Geometry: final body of the model. Coordinates: model frame, mm. Face numbers are marked on the shaded views. A direction names the side the tool comes from. Give positions to 0.01 mm unless a question says otherwise; leave off trailing zeros. Order: outer loops, then holes, each group sorted by start corner. A loop starts at its lowest first (then second) coordinate and runs counter-clockwise, first axis right, second up. Notation, with made-up numbers: (62.25, 49.5) - (112.25, 49.5) arc R12 cw to (112.25, 55.5) - close; hole circle Ø9 at (58.25, -20). An arc over 180 degrees is marked (long way). Use one line per item in the form item = value.
from build123d import *

# Parameters (mm, degrees)
SKETCH1_W           = 30
SKETCH1_H           = 85
BOSS_EXTRUDE1_DEPTH = 10
SKETCH2_W           = 30
SKETCH2_H           = 15
BOSS_EXTRUDE2_DEPTH = 2.5
SKETCH3_W           = 3
SKETCH3_H           = 15
BOSS_EXTRUDE3_DEPTH = 3


with BuildPart() as part:
    # Sketch1 → Boss-Extrude1 (new body)
    with BuildSketch(Plane.XY):
        with Locations((15, 42.5)):
            Rectangle(SKETCH1_W, SKETCH1_H)
    extrude(amount=BOSS_EXTRUDE1_DEPTH)

    # Sketch2 → Boss-Extrude2 (add)
    with BuildSketch(Plane.XY.offset(10)):
        with Locations((15, 62.5)):
            Rectangle(SKETCH2_W, SKETCH2_H)
        with Locations((15, 22.5)):
            Rectangle(SKETCH2_W, SKETCH2_H)
    extrude(amount=BOSS_EXTRUDE2_DEPTH)

    # Sketch3 → Boss-Extrude3 (add)
    with BuildSketch(Plane.XY.offset(12.5)):
        with Locations((28.5, 62.5)):
            Rectangle(SKETCH3_W, SKETCH3_H)
        with Locations((28.5, 22.5)):
            Rectangle(SKETCH3_W, SKETCH3_H)
        with Locations((1.5, 22.5)):
            Rectangle(SKETCH3_W, SKETCH3_H)
        with Locations((1.5, 62.5)):
            Rectangle(SKETCH3_W, SKETCH3_H)
    extrude(amount=BOSS_EXTRUDE3_DEPTH)


solid = part.part
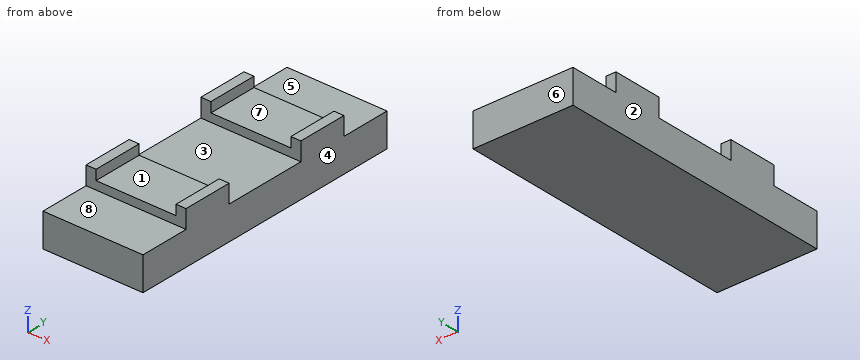
(1) Reachability of the marked faces 4, 5, 6, 7 and 8 from +Z, -Z, +X, -X, +Y, -Y: full face, straight path, thin tool, end or side. Return the list, or none.
Computed values:
face_4 = +Z, -Z, +X, +Y, -Y
face_5 = +Z, +X, -X, +Y
face_6 = +Z, -Z, +X, -X, +Y
face_7 = +Z, +Y, -Y
face_8 = +Z, +X, -X, -Y
(2) Cut plane B-B on y = 56. Output: boundary loops of the cut face in (x, z).
Computed values:
outline = (0, 0) - (30, 0) - (30, 15.5) - (27, 15.5) - (27, 12.5) - (3, 12.5) - (3, 15.5) - (0, 15.5) - close
(3) Pull-direction query (X, two-part tool) for the marked faces 1, 2 and 3; classes: released by +X, released by -X, zero draft, split by the parting line, or undercut.
Computed values:
face_1 = undercut
face_2 = released by -X
face_3 = zero draft
(4) Cut plane D-D on x = 28. Output: boundary loops of the cut face in (y, z), plus the area to 4 significant figures.
Computed values:
outline = (0, 0) - (85, 0) - (85, 10) - (70, 10) - (70, 15.5) - (55, 15.5) - (55, 10) - (30, 10) - (30, 15.5) - (15, 15.5) - (15, 10) - (0, 10) - close
area = 1,015 mm²
(5) Cut plane C-C on x = 6.5. Output: boundary loops of the cut face in (y, z).
Computed values:
outline = (0, 0) - (85, 0) - (85, 10) - (70, 10) - (70, 12.5) - (55, 12.5) - (55, 10) - (30, 10) - (30, 12.5) - (15, 12.5) - (15, 10) - (0, 10) - close
(6) Cut plane A-A on z = 14.25. Output: boundary loops of the cut face in (x, y).
Computed values:
outline = (0, 15) - (3, 15) - (3, 30) - (0, 30) - close; (0, 55) - (3, 55) - (3, 70) - (0, 70) - close; (27, 15) - (30, 15) - (30, 30) - (27, 30) - close; (27, 55) - (30, 55) - (30, 70) - (27, 70) - close
(7) Contact query for flat-ended pins moving along their axis: pin 1 Ø16.5 at (x, y) = (17, 24) entering from +Z; pin 2 Ø4.5 at (x, z) = (16, 12.5) entering from -Y; pin 3 Ø1.5 at (x, y) = (21, 14) entering from +Z. Output: stop coordinate, or through.
Computed values:
pin_1 = 12.5
pin_2 = 15
pin_3 = 10
(8) Ray query, line 1 along Y through (x, z) = (14, 12); line 2 along Z through (x, y) = (11, 21.5); line 3 along Z through (x, y) = (17.25, 80). Return the intervals inside material, ascending.
Computed values:
line_1 = 15 to 30, 55 to 70
line_2 = 0 to 12.5
line_3 = 0 to 10
